The listing builds one solid part. Answer for the finished solid, in the listing's coordinates (mm). A direction names the side the tool comes from. Give positions to 0.01 mm unless a question says otherwise; leave off trailing zeros. Write each loop counter-clockwise with the first axis right and the second up, starting at its lowest first coordinate (ties: lowest second). Pieces come first, ordered by that corner, then holes. Notation, with made-up numbers: (66, 9.25) -> (95, 9.25) arc R20 cw to (95, 46.25) -> close; hole circle Ø11 at (-39.75, 1). An arc over 180 degrees is marked (long way). Put each result on its own line as item: value. Start each with the question number.
1) A cutting plane is placed at A-A (y = 0). Write down the section's boundary in (x, z) (3 decimals).
2) Find the intervals of material crossed by line 1 along Y through (x, z) = (0, 17.5); line 2 along Z through (x, y) = (-19.5, 22.5); line 3 along Y through (x, z) = (0, 1.95) (3 decimals), in increasing order. Write a range as from..to.
3) A cutting plane is placed at C-C (z = 11.75). Write down the section's boundary in (x, y), then the cut area to 3 significant figures.
4) For faces 1 (the cylindrical face through (-7.709, -34.714, 13.81)), 2 (the flat face through (0, -7, 0)), determine the directions among +Z, -Z, +X, -X, +Y, -Y from which every point of the face is accessible in a straight line to the end or side of a thin tool.
5) Flat-ended cylindrical pins translate along their axes: pin 1 Ø4 at (y, z) = (25.5, 11.5) entering from -X; pin 2 Ø12 at (y, z) = (27, 20.5) entering from +X; pin 3 Ø4 at (y, z) = (-13.5, 6.5) entering from +X; pin 4 Ø12 at (x, y) = (26, -3.5) entering from -Z. Find the tip coordinate at first contact, or state that the pin passes through.
from build123d import *

# Parameters (mm, degrees)
F0_R     = 38.1
F1_DEPTH = 25.4
F2_T     = -2.54
F3_SIZE  = 2.54
F5_D     = 6.35


with BuildPart() as f1:
    # F0 (on Top) → F1 (new body)
    with BuildSketch(Plane.XY):
        Circle(F0_R)
    extrude(amount=F1_DEPTH)

    # F2
    f2_openings = [f1.faces().sort_by_distance(p)[0] for p in [
        (0, 0, 25.4),
    ]]
    offset(amount=F2_T, openings=f2_openings)

    # F3
    f3_edges = [f1.edges().sort_by_distance(p)[0] for p in [
        (-38.1, 0, 0),
    ]]
    chamfer(f3_edges, length=F3_SIZE)

    # F5 (through all)
    with Locations(Plane(origin=(0, 0, 0), x_dir=(1, 0, 0), z_dir=(0, 0, -1))):
        with Locations((0, 0)):
            Hole(F5_D / 2)


solid = f1.part
Reply:
1. outline: (-38.1, 2.54) -> (-35.56, 0) -> (-3.175, 0) -> (-3.175, 2.54) -> (-35.56, 2.54) -> (-35.56, 25.4) -> (-38.1, 25.4) -> close; (3.175, 0) -> (35.56, 0) -> (38.1, 2.54) -> (38.1, 25.4) -> (35.56, 25.4) -> (35.56, 2.54) -> (3.175, 2.54) -> close
2. line 1: y = -38.1..-35.56, 35.56..38.1
2. line 2: z = 0..2.54
2. line 3: y = -37.51..-3.175, 3.175..37.51
3. outline: circle Ø76.2 at (0, 0); hole circle Ø71.12 at (0, 0)
3. area: 588 mm2
4. face 1: +Z
4. face 2: -Z, +X, -X, +Y, -Y
5. pin 1: stops at x = -29.99
5. pin 2: stops at x = 31.79
5. pin 3: stops at x = 36.32
5. pin 4: stops at z = 0
